from build123d import *

# Parameters (mm, degrees)
F0_W      = 40
F0_H      = 23
F0_W_2    = 0.3508773884
F0_H_2    = 0.3508765315
F1_DEPTH  = 35
F2_DEPTH  = 3
F3_R      = 1
F4_R      = 1
F8_DEPTH  = 6
F10_R     = 3
F11_DEPTH = 17


# Not quite as in the source:
# - two fillets or chamfers of one size are made in one step


with BuildPart() as f1:
    # F0 (on Front) → F1 (new body)
    with BuildSketch(Plane.XZ):
        with Locations((-11.8218250573, 18.8361621085)):
            Rectangle(F0_W, F0_H)
        with Locations((-10.2428785232, 26.8098455974)):
            Rectangle(F0_W_2, F0_H_2, mode=Mode.SUBTRACT)
    extrude(amount=F1_DEPTH)

    # F2 (add): a face of the model
    f2_faces = [f1.faces().sort_by_distance(p)[0] for p in [
        (-31.8218250573, -17.5, 18.8361621085),
    ]]
    extrude(f2_faces, amount=F2_DEPTH)

    # F3
    f3_edges = [f1.edges().sort_by_distance(p)[0] for p in [
        (-13.321825, -35, 30.336162),
    ]]
    fillet(f3_edges, radius=F3_R)

    # F4
    f4_edges = [f1.edges().sort_by_distance(p)[0] for p in [
        (-13.321825, -35, 7.336162),
        (8.178175, -17, 30.336162),
        (8.178175, -17.5, 7.336162),
        (-13.321825, 0, 30.336162),
        (-13.321825, 0, 7.336162),
        (-34.821825, -17, 30.336162),
        (8.178175, -34.707107, 30.043269),
        (8.178175, 0, 18.836162),
        (8.178175, -35, 18.336162),
        (-34.821825, -34.707107, 30.043269),
        (-34.821825, 0, 18.836162),
        (-34.821825, -35, 18.336162),
        (-34.821825, -17.5, 7.336162),
    ]]
    fillet(f4_edges, radius=F4_R)

    # F7 (on face) → F8 (cut)
    with BuildSketch(Plane(origin=(0, 0, 7.3361621085), x_dir=(1, 0, 0), z_dir=(0, 0, -1))):
        Polygon((-15.4886602973, 23.0950714957), (-19.2507167286, 18.4210013842), (-17.0838814885, 12.8259298884), (-11.1549898172, 11.9049285043), (-7.3929333859, 16.5789986158), (-9.559768626, 22.1740701116), align=None)
    extrude(amount=-F8_DEPTH, mode=Mode.SUBTRACT)

    # F10 (on face) → F11 (cut, through all)
    with BuildSketch(Plane(origin=(0, 0, 13.3361621085), x_dir=(1, 0, 0), z_dir=(0, 0, -1))):
        with Locations((-13.3786574006, 17.5000000745)):
            Circle(F10_R)
    extrude(amount=-F11_DEPTH, mode=Mode.SUBTRACT)


solid = f1.part
Can you work these out from the model? Positions are in its coordinate system, mm. A direction names the side the tool comes from. Give positions to 0.01 mm unless a question says otherwise; leave off trailing zeros. Write each loop counter-clockwise with the first axis right and the second up, starting at its lowest first coordinate (ties: lowest second). Pieces come first, ordered by that corner, then holes. Notation, with made-up numbers: (-30, 6.5) -> (-10, 6.5) arc R18 cw to (-10, 30.5) -> close; hole circle Ø11 at (46, 75.5). An arc over 180 degrees is marked (long way). Answer as a JSON object with one key per item and string values. Group by question number.
Item 1: Suppose I cut it at B-B (y = -19). Please give me the cut outline in (x, z).
Item 2: Please list where these lines run through material, in increasing order: line 1 (X direction, y = -17.5, z = 23.75); line 2 (Y direction, x = -11.5, z = 27.5); line 3 (Z direction, x = -12, y = -14). Write a range as [from, to].
Item 3: Suppose I cut it at A-A (z = 11.25). Please give me the cut outline in (x, y).
Item 4: We'd pull the mould along Y, two halves only. Please class faces 1 (the face through (-11, -15, 13.336)), 2 (the face through (-13, 0, 19)), 3 (the face through (7.89, -17.73, 30.04)): +Y half, -Y half, draft (parallel to the pull), parting line (faces both ways), or undercut.
Item 5: Suppose I cut it at D-D (y = -15). Please give me the cut outline in (x, z), plus the area to 3 significant figures.
Item 6: For faces 4 (the face through (-9.3, -14.21, 10.29)), 5 (the face through (-34.5, -17.7, 7.6)), which set-ups out of +Z, -Z, +X, -X, +Y, -Y let a thin tool reach every point of the face, with its end or its side?
Item 7: I'm going to push a flat-ended pin straight in: P1, Ø1.5, axis at x = -12, y = -15.5, coming from the -Z side. Where does the tip first touch, or does it pass through?
Item 8: Suppose I cut it at C-C (z = 19.5). Please give me the cut outline in (x, y), plus the area to 3 significant figures.
Findings:
{
 "1": {"outline": "(-34.82, 8.34) arc R1 ccw to (-33.82, 7.34) -> (-18.78, 7.34) -> (-18.78, 13.34) -> (-15.98, 13.34) -> (-15.98, 30.34) -> (-33.82, 30.34) arc R1 ccw to (-34.82, 29.34) -> close; (-10.78, 13.34) -> (-8.33, 13.34) -> (-8.33, 7.34) -> (7.18, 7.34) arc R1 ccw to (8.18, 8.34) -> (8.18, 29.34) arc R1 ccw to (7.18, 30.34) -> (-10.78, 30.34) -> close; hole (-10.42, 26.63) -> (-10.07, 26.63) -> (-10.07, 26.99) -> (-10.42, 26.99) -> close"},
 "2": {"line 1": "x = [-34.82, -16.38], [-10.38, 8.18]", "line 2": "y = [-35, -19.84], [-15.16, 0]", "line 3": "z = [13.34, 30.34]"},
 "3": {"outline": "(-34.82, -34) arc R1 ccw to (-33.82, -35) -> (7.18, -35) arc R1 ccw to (8.18, -34) -> (8.18, -1) arc R1 ccw to (7.18, 0) -> (-33.82, 0) arc R1 ccw to (-34.82, -1) -> close; hole (-19.25, -18.42) -> (-15.49, -23.1) -> (-9.56, -22.17) -> (-7.39, -16.58) -> (-11.15, -11.9) -> (-17.08, -12.83) -> close"},
 "4": {"face 1": "undercut", "face 2": "+Y half", "face 3": "draft"},
 "5": {"outline": "(-34.82, 8.34) arc R1 ccw to (-33.82, 7.34) -> (-17.93, 7.34) -> (-17.93, 13.34) -> (-15.04, 13.34) -> (-15.04, 30.34) -> (-33.82, 30.34) arc R1 ccw to (-34.82, 29.34) -> close; (-11.72, 13.34) -> (-8.66, 13.34) -> (-8.66, 7.34) -> (7.18, 7.34) arc R1 ccw to (8.18, 8.34) -> (8.18, 29.34) arc R1 ccw to (7.18, 30.34) -> (-11.72, 30.34) -> close; hole (-10.42, 26.63) -> (-10.07, 26.63) -> (-10.07, 26.99) -> (-10.42, 26.99) -> close", "area": "876 mm²"},
 "6": {"face 4": "-Z", "face 5": "-Z, -X, +Y, -Y"},
 "7": {"P1": "stops at z = 13.34"},
 "8": {"outline": "(-34.82, -34) arc R1 ccw to (-33.82, -35) -> (7.18, -35) arc R1 ccw to (8.18, -34) -> (8.18, -1) arc R1 ccw to (7.18, 0) -> (-33.82, 0) arc R1 ccw to (-34.82, -1) -> close; hole circle Ø6 at (-13.38, -17.5)", "area": "1,480 mm²"}
}
